from build123d import *

# Parameters (mm, degrees)
CROQUIS1_W              = 50
CROQUIS1_H              = 100
CROQUIS1_R              = 20
SALIENTE_EXTRUIR1_DEPTH = 50
CROQUIS2_R              = 20
SALIENTE_EXTRUIR2_DEPTH = 75


with BuildPart() as part:
    # Croquis1 → Saliente-Extruir1 (new body)
    with BuildSketch(Plane(origin=(0, 0, 0), x_dir=(1, 0, 0), z_dir=(0, 1, 0))):
        with Locations((0, -10)):
            Rectangle(CROQUIS1_W, CROQUIS1_H)
        Circle(CROQUIS1_R, mode=Mode.SUBTRACT)
    extrude(amount=SALIENTE_EXTRUIR1_DEPTH)

    # Croquis2 → Saliente-Extruir2 (add)
    with BuildSketch(Plane(origin=(0, 0, -40), x_dir=(-1, 0, 0), z_dir=(0, 0, -1))):
        with Locations((0, 25)):
            Circle(CROQUIS2_R)
    extrude(amount=SALIENTE_EXTRUIR2_DEPTH)


solid = part.part
Check sheet for the modelled part. Datum: model origin and axes. Units: mm. A direction names the side the tool comes from. Give positions to 0.01 mm unless a question says otherwise; leave off trailing zeros. Write each loop counter-clockwise with the first axis right and the second up, starting at its lowest first coordinate (ties: lowest second). Pieces come first, ordered by that corner, then holes. Notation, with made-up numbers: (-9.5, 33) -> (31.5, 33) arc R19 ccw to (31.5, 64) -> close; hole circle Ø11 at (69.5, 59). An arc over 180 degrees is marked (long way). One line per item, written item: value. Start each with the question number.
Item 1: Tool access check on faces 1 (the cylindrical face through (4.336, 5.476, -76.975)), 2 (the flat face through (-0.3, 0, 20.4)). Record the directions out of +Z, -Z, +X, -X, +Y, -Y that give a thin tool (end or side, any length) a straight path to the whole face; none if there is none.
Item 2: Section check C-C on y = 13. Record the cut outline in (x, z).
Item 3: Section check D-D on y = 25. Record the cut outline in (x, z).
Item 4: Section check B-B on x = 0. Record the cut outline in (y, z), then the cut area to 3 significant figures.
Item 5: Section check A-A on z = 0. Record the cut outline in (x, y).
Item 6: Draft check along X on faces 3 (the cylindrical face through (-4.336, 24.65, 19.524)), 4 (the flat face through (-25, 25, 11)), 5 (the flat face through (0, 25, 60)). Enter one of: +X half, -X half, draft (parallel to the pull), parting line (faces both ways), or undercut.
Item 7: Gauge pin test, flat ends, axial feed: pin 1 (4 mm diameter, centred on y = 33.5, z = -76, fed in from -X); pin 2 (12 mm diameter, centred on y = 5, z = -78, fed in from -X); pin 3 (1 mm diameter, centred on x = 0.5, z = -69.5, fed in from -Y). Record the tip position at first contact, or that the pin passes through.
Item 8: Material ranges on probe 1 along Z at (x, y) = (0, 40); probe 2 along X at (y, z) = (15, 0); probe 3 along Z at (x, y) = (-15.5, 22), recorded low to high. Write a range as from..to.
Results list:
1. face 1: -Z
1. face 2: +Z, -Z, +X, -X, -Y
2. outline: (-25, -40) -> (-16, -40) -> (-16, -115) -> (16, -115) -> (16, -40) -> (25, -40) -> (25, 60) -> (-25, 60) -> close; hole circle Ø40 at (0, 0)
3. outline: (-25, -40) -> (-20, -40) -> (-20, -115) -> (20, -115) -> (20, -40) -> (25, -40) -> (25, 60) -> (-25, 60) -> close; hole circle Ø40 at (0, 0)
4. outline: (0, -40) -> (5, -40) -> (5, -115) -> (45, -115) -> (45, -40) -> (50, -40) -> (50, -20) -> (0, -20) -> close; (0, 20) -> (50, 20) -> (50, 60) -> (0, 60) -> close
4. area: 6,000 mm²
5. outline: (-25, 0) -> (-20, 0) -> (-20, 50) -> (-25, 50) -> close; (20, 0) -> (25, 0) -> (25, 50) -> (20, 50) -> close
6. face 3: undercut
6. face 4: -X half
6. face 5: draft
7. pin 1: x = -18.91
7. pin 2: x = -14.28
7. pin 3: y = 5
8. probe 1: -115..-20, 20..60
8. probe 2: -25..-20, 20..25
8. probe 3: -115..-12.64, 12.64..60
